```python
from build123d import *

# Parameters (mm, degrees)
SKETCH1_W             = 50
SKETCH1_H             = 64
SKETCH1_W_2           = 29.2
SKETCH1_H_2           = 40
BOSS_EXTRUDE1_DEPTH   = 15
SKETCH3_W             = 7
SKETCH3_H             = 11.1
SKETCH4_R             = 9.5
CUT_EXTRUDE2_DEPTH    = 51
SKETCH5_R             = 4
CUT_EXTRUDE3_DEPTH    = 65
SKETCH8_R             = 2.15
CUT_EXTRUDE6_DEPTH    = 16
FILLET1_R             = 20
CHAMFER1_SIZE         = 3
CHAMFER1_SIZE2        = 1.732050808
CHAMFER1_PART_2_SIZE  = 3
CHAMFER1_PART_2_SIZE2 = 1.732050808
SKETCH9_W             = 12
SKETCH9_H             = 3


with BuildPart() as part:
    # Sketch1 → Boss-Extrude1 (new body)
    with BuildSketch(Plane(origin=(0, 0, 0), x_dir=(1, 0, 0), z_dir=(0, 1, 0))):
        Rectangle(SKETCH1_W, SKETCH1_H)
        Rectangle(SKETCH1_W_2, SKETCH1_H_2, mode=Mode.SUBTRACT)
    extrude(amount=BOSS_EXTRUDE1_DEPTH)

    # Sketch3 → Cut-Revolve1 (revolve, cut)
    with BuildSketch(Plane(origin=(0, 15, 0), x_dir=(1, 0, 0), z_dir=(0, 1, 0))):
        with Locations((18.1, -5.55)):
            Rectangle(SKETCH3_W, SKETCH3_H)
        with Locations((-18.1, -5.55)):
            Rectangle(SKETCH3_W, SKETCH3_H)
    revolve(axis=Axis((14.6, 15, 0), (1, 0, 0)), mode=Mode.SUBTRACT)

    # Sketch4 → Cut-Extrude2 (cut, through all)
    with BuildSketch(Plane(origin=(25, 0, 0), x_dir=(0, 0, -1), z_dir=(1, 0, 0))):
        with Locations((0, 15)):
            Circle(SKETCH4_R)
    extrude(amount=-CUT_EXTRUDE2_DEPTH, mode=Mode.SUBTRACT)

    # Sketch5 → Cut-Extrude3 (cut, through all)
    with BuildSketch(Plane.XY.offset(32)):
        with Locations((0, 15)):
            Circle(SKETCH5_R)
    extrude(amount=-CUT_EXTRUDE3_DEPTH, mode=Mode.SUBTRACT)

    # Sketch8 → Cut-Extrude6 (cut, through all)
    with BuildSketch(Plane(origin=(0, 15, 0), x_dir=(1, 0, 0), z_dir=(0, 1, 0))):
        with Locations(Location((18, 16.5, 0), (0, 0, 270))):  # turned: the seam where the file's is
            Circle(SKETCH8_R)
        with Locations(Location((18, -16.5, 0), (0, 0, 270))):  # turned: the seam where the file's is
            Circle(SKETCH8_R)
        with Locations(Location((-18, -16.5, 0), (0, 0, 270))):  # turned: the seam where the file's is
            Circle(SKETCH8_R)
        with Locations(Location((-18, 16.5, 0), (0, 0, 270))):  # turned: the seam where the file's is
            Circle(SKETCH8_R)
        with Locations(Location((9, -27, 0), (0, 0, 270))):  # turned: the seam where the file's is
            Circle(SKETCH8_R)
        with Locations(Location((-9, -27, 0), (0, 0, 270))):  # turned: the seam where the file's is
            Circle(SKETCH8_R)
        with Locations(Location((-9, 27, 0), (0, 0, 270))):  # turned: the seam where the file's is
            Circle(SKETCH8_R)
        with Locations(Location((9, 27, 0), (0, 0, 270))):  # turned: the seam where the file's is
            Circle(SKETCH8_R)
    extrude(amount=-CUT_EXTRUDE6_DEPTH, mode=Mode.SUBTRACT)

    # Fillet1
    fillet1_edges = [part.edges().sort_by_distance(p)[0] for p in [
        (-25, 7.5, -32),
        (25, 7.5, -32),
        (25, 7.5, 32),
        (-25, 7.5, 32),
    ]]
    fillet(fillet1_edges, radius=FILLET1_R)

    # Chamfer1
    chamfer1_edges = [part.edges().sort_by_distance(p)[0] for p in [
        (14.6, 3.9, 0),
    ]]
    chamfer1_side = [part.faces().sort_by_distance(p)[0] for p in [
        (14.6, 0.427200187, 0),
    ]]
    chamfer(chamfer1_edges, length=CHAMFER1_SIZE, length2=CHAMFER1_SIZE2, reference=chamfer1_side[0])

    # Chamfer1 part 2
    chamfer1_part_2_edges = [part.edges().sort_by_distance(p)[0] for p in [
        (-14.6, 3.9, 0),
    ]]
    chamfer1_part_2_side = [part.faces().sort_by_distance(p)[0] for p in [
        (-14.6, 0.427200187, 0),
    ]]
    chamfer(chamfer1_part_2_edges, length=CHAMFER1_PART_2_SIZE, length2=CHAMFER1_PART_2_SIZE2, reference=chamfer1_part_2_side[0])

    # Sketch9 → Cut-Revolve2 (revolve, cut)
    with BuildSketch(Plane(origin=(0, 15, 0), x_dir=(1, 0, 0), z_dir=(0, 1, 0))):
        with Locations((-6, -21.5)):
            Rectangle(SKETCH9_W, SKETCH9_H)
        with Locations((-6, 21.5)):
            Rectangle(SKETCH9_W, SKETCH9_H)
    revolve(axis=Axis((0, 15, -29.871415895), (0, 0, 1)), mode=Mode.SUBTRACT)


solid = part.part
```
Could you check a few things on this model? Use its own coordinates, in mm. A direction names the side the tool comes from. Round coordinates to 2 decimals unless told otherwise and drop trailing zeros. Loops run counter-clockwise (first coordinate to the right, second up) from the corner with the lowest first, then second, coordinate; pieces in that order, holes last. Notation, with made-up numbers: (74.5, -0.5) - (109.5, -0.5) arc R9 cw to (109.5, 7.5) - close; hole circle Ø3 at (1, 36). An arc over 180 degrees is marked (long way). Use CSV: the item, a comma, the result in double quotes.
Item 1: If we section it at D-D on x = -2: List the corners of the cut face in (y, z) for me, then the cut area to 3 significant figures.
Here are the results:
outline,"(0, -32) - (11.54, -32) - (11.54, -23) - (3.17, -23) - (3.17, -20) - (0, -20) - close; (0, 20) - (3.17, 20) - (3.17, 23) - (11.54, 23) - (11.54, 32) - (0, 32) - close"
area,"227 mm²"
Item 2: If we section it at C-C on x = -17: List the corners of the cut face in (y, z) for me, then the cut area to 3 significant figures.
Here are the results:
outline,"(0, -28) - (15, -28) - (15, -18.4) - (0, -18.4) - close; (0, -14.6) - (15, -14.6) - (15, -11.1) arc R11.1 cw to (15, 11.1) - (15, 14.6) - (0, 14.6) - close; (0, 18.4) - (15, 18.4) - (15, 28) - (0, 28) - close"
area,"532 mm²"
Item 3: I need wall thicknesses on L1, parallel to X at y = 1.75, z = -15.5; L2, parallel to X at y = 10, z = 8.5; L3, parallel to Z at x = -2, y = 8.75. Which ranges of each line are inside material? Lowest first, please. Write a range as [from, to].
Here are the results:
L1,"x = [-24.69, -19.9], [-16.1, -14.6], [14.6, 16.1], [19.9, 24.69]"
L2,"x = [-25, -21.6], [21.6, 25]"
L3,"z = [-32, -23], [23, 32]"
Item 4: Will these pins go through, and if not, where does the flat tip stop? pin 1 (3 mm diameter, centred on y = 10, z = -15.5, fed in from -X); pin 2 (3.5 mm diameter, centred on x = -18, z = 16.5, fed in from +Y); pin 3 (1 mm diameter, centred on y = 6.5, z = 16, fed in from -X); pin 4 (6 mm diameter, centred on y = 8.5, z = -25.5, fed in from +X).
Here are the results:
pin 1,"stops at x = -24.9"
pin 2,"passes through"
pin 3,"stops at x = -24.69"
pin 4,"stops at x = 22.02"
Item 5: If we mould it in two halves opening along X, with no side actions, what happens to faces 1 (the flat face through (14, 15, 23)), 2 (the cylindrical face through (-19.297, 7.605, -25.986)), 3 (the cylindrical face through (-20.1, 7.6, 16.03))? For each: pulls with the +X half, pulls with the -X half, needs draft (parallel to the pull), parting line crosses it, or undercut.
Here are the results:
face 1,"needs draft"
face 2,"pulls with the -X half"
face 3,"undercut"
Item 6: For faces 4 (the cylindrical face through (-18.9, 3.9, 0.2)), 5 (the flat face through (-25, 4, 0)), which set-ups out of +Z, -Z, +X, -X, +Y, -Y let a thin tool reach every point of the face, with its end or its side?
Here are the results:
face 4,"+Y"
face 5,"+Z, -Z, -X, +Y, -Y"
Item 7: If we section it at B-B on z = 16.5: List the corners of the cut face in (x, y) for me.
Here are the results:
outline,"(-24.49, 0) - (-20.15, 0) - (-20.15, 15) - (-24.49, 15) - close; (-15.85, 0) - (-14.6, 0) - (-14.6, 15) - (-15.85, 15) - close; (14.6, 0) - (15.85, 0) - (15.85, 15) - (14.6, 15) - close; (20.15, 0) - (24.49, 0) - (24.49, 15) - (20.15, 15) - close"
Item 8: If we section it at A-A on x = -9: List the corners of the cut face in (y, z) for me, then the cut area to 3 significant figures.
Here are the results:
outline,"(0, -31.6) - (15, -31.6) - (15, -29.15) - (0, -29.15) - close; (0, -24.85) - (15, -24.85) - (15, -23) - (7.06, -23) - (7.06, -20) - (0, -20) - close; (0, 20) - (7.06, 20) - (7.06, 23) - (15, 23) - (15, 24.85) - (0, 24.85) - close; (0, 29.15) - (15, 29.15) - (15, 31.6) - (0, 31.6) - close"
area,"171 mm²"
